Geometry: final body of the model. Coordinates: model frame, mm. A direction names the side the tool comes from. Give positions to 0.01 mm unless a question says otherwise; leave off trailing zeros. Write each loop counter-clockwise with the first axis right and the second up, starting at its lowest first coordinate (ties: lowest second). Pieces come first, ordered by that corner, then holes. Notation, with made-up numbers: M 5.5,88 L 51.5,88 A30 cw 51.5,113 Z; hole C -31.75,13.25 d7. An arc over 180 degrees is marked long. Answer as a JSON object with one key per item and string values.
from build123d import *

# Parameters (mm, degrees)
EXTRUDE_1_DEPTH = 2
SKETCH_3_W      = 3.4
SKETCH_3_H      = 17
EXTRUDE_2_DEPTH = 10


with BuildPart() as part:
    # 스케치1 → 보스-돌출1 (new body)
    with BuildSketch(Plane.XY):
        with BuildLine():
            Line((-0.518908087, 12.196403379), (34.938840058, 25.5))
            Line((34.938840058, 25.5), (34.938840058, 8.5))
            Line((34.938840058, 8.5), (0.107473336, 1.965709515))
            ThreePointArc((0.107473336, 1.965709515), (-1.52376373, 0), (0.107473336, -1.965709515))
            Line((0.107473336, -1.965709515), (34.938840058, -8.5))
            Line((34.938840058, -8.5), (34.938840058, -25.5))
            Line((34.938840058, -25.5), (-0.518908087, -12.196403379))
            ThreePointArc((-0.518908087, -12.196403379), (-10.539851544, -9.431582272), (-20.893387075, -8.5))
            Line((-20.893387075, -8.5), (-61.061159942, -8.5))
            Line((-61.061159942, -8.5), (-61.061159942, 8.5))
            Line((-61.061159942, 8.5), (-20.893387075, 8.5))
            ThreePointArc((-20.893387075, 8.5), (-10.539851544, 9.431582272), (-0.518908087, 12.196403379))
        make_face()
    extrude(amount=EXTRUDE_1_DEPTH)

    # 스케치3 → 보스-돌출2 (add)
    with BuildSketch(Plane(origin=(0, 0, 0), x_dir=(-1, 0, 0), z_dir=(0, 0, -1))):
        Polygon((-34.938840058, 25.5), (-34.938840058, 8.5), (-30.348840058, 8.5), (-30.348840058, 23.77785148), align=None)
        Polygon((-34.938840058, -8.5), (-34.938840058, -25.5), (-30.348840058, -23.77785148), (-30.348840058, -8.5), align=None)
        with Locations((59.361159942, 0)):
            Rectangle(SKETCH_3_W, SKETCH_3_H)
    extrude(amount=EXTRUDE_2_DEPTH)


solid = part.part
1) Cut plane A-A on z = -4. Return loops of the section in (x, y).
Geometry check:
{"outline": "M -61.06,-8.5 L -57.66,-8.5 L -57.66,8.5 L -61.06,8.5 Z; M 30.35,-23.78 L 34.94,-25.5 L 34.94,-8.5 L 30.35,-8.5 Z; M 30.35,8.5 L 34.94,8.5 L 34.94,25.5 L 30.35,23.78 Z"}
2) Contact query for flat-ended pins moving along their axis: P1, Ø6, axis at x = -46.5, z = -4.5, coming from the +Y side; P2, Ø4, axis at x = 18, y = -13, coming from the -Z side; P3, Ø1.5, axis at x = 25, z = 0, coming from the +Y side; P4, Ø6, axis at x = 13, z = -2, coming from the -Y side. Output: stop coordinate, or through.
Geometry check:
{"P1": "passes through", "P2": "stops at z = 0", "P3": "stops at y = 22.05", "P4": "stops at y = -18.11"}
3) Line query: line 1 (Z direction, x = 18.5, y = 11); line 2 (X direction, y = 12.5, z = -8.25); line 3 (X direction, y = 6, z = -1). Output: solid intervals per line, ascending. Write a range as from..to.
Geometry check:
{"line 1": "z = 0..2", "line 2": "x = 30.35..34.94", "line 3": "x = -61.06..-57.66"}
4) Cut plane B-B on x = 18. Return loops of the section in (y, z).
Geometry check:
{"outline": "M -19.14,0 L -5.32,0 L -5.32,2 L -19.14,2 Z; M 5.32,0 L 19.14,0 L 19.14,2 L 5.32,2 Z"}
5) Cut plane D-D on x = -39. Return loops of the section in (y, z).
Geometry check:
{"outline": "M -8.5,0 L 8.5,0 L 8.5,2 L -8.5,2 Z"}
6) Pull-direction query (Y, two-part tool) for faces 4 (the flat face through (17.279, -5.187, 0.986)), 5 (the cylindrical face through (-10.396, -9.458, 0.986)), 6 (the flat face through (34.939, 17, -4)); classes: pulls with the +Y half, pulls with the -Y half, needs draft (parallel to the pull), parting line crosses it, or undercut.
Geometry check:
{"face 4": "undercut", "face 5": "pulls with the -Y half", "face 6": "needs draft"}
7) Cut plane C-C on y = 5. Return loops of the section in (x, z), and give its area (3 significant figures).
Geometry check:
{"outline": "M -61.06,-10 L -57.66,-10 L -57.66,0 L 16.28,0 L 16.28,2 L -61.06,2 Z", "area": "189 mm2"}
8) Set-up query: faces 1 (the flat face through (-57.661, 0, -5)), 2 (the flat face through (-45.3, -8.5, 0.4)), 3 (the flat face through (-47, 8.5, 0.4)). Return all of +Z, -Z, +X, -X, +Y, -Y with unobstructed straight access to the full face (end or side cutting, diameter ignored); none if empty.
Geometry check:
{"face 1": "-Z, +X, +Y, -Y", "face 2": "+Z, -Z, -X, -Y", "face 3": "+Z, -Z, -X, +Y"}
